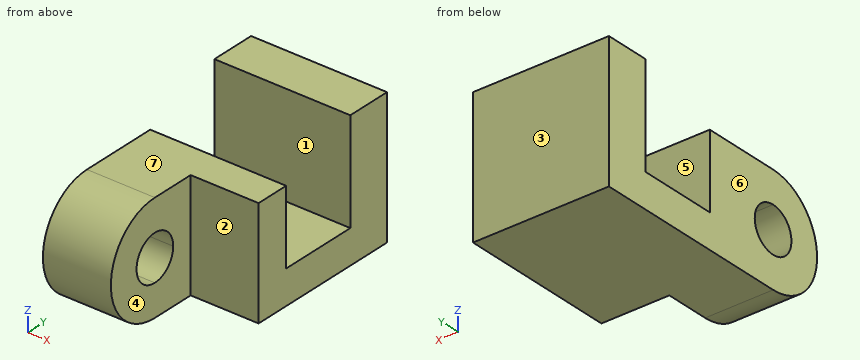
from build123d import *

# Parameters (mm, degrees)
F0_W      = 700
F0_H      = 600
F1_DEPTH  = 600
F3_DEPTH  = 600.001
F4_W      = 150
F4_H      = 120
F5_DEPTH  = 600.001
F6_W      = 300
F6_H      = 480
F7_DEPTH  = 195
F9_DEPTH  = 300
F11_DEPTH = 300.001


with BuildPart() as f1:
    # F0 (on Right) → F1 (new body)
    with BuildSketch(Plane.YZ):
        Rectangle(F0_W, F0_H)
    extrude(amount=F1_DEPTH)

    # F2 (on face) → F3 (cut, through all)
    with BuildSketch(Plane.YZ.offset(600)):
        Polygon((150, -150), (150, 300), (-200, 300), (-200, -150), (0, -150), align=None)
    extrude(amount=-F3_DEPTH, mode=Mode.SUBTRACT)

    # F4 (on face) → F5 (cut, through all)
    with BuildSketch(Plane.YZ.offset(600)):
        with Locations((-275, 240)):
            Rectangle(F4_W, F4_H)
    extrude(amount=-F5_DEPTH, mode=Mode.SUBTRACT)

    # F6 (on face) → F7 (join)
    with BuildSketch(Plane.XZ.offset(350)):
        with Locations((150, -60)):
            Rectangle(F6_W, F6_H)
    extrude(amount=F7_DEPTH)

    # F8 (on face) → F9 (join)
    with BuildSketch(Plane(origin=(0, 0, 0), x_dir=(0, -1, 0), z_dir=(-1, 0, 0))):
        with BuildLine():
            ThreePointArc((545, -300), (714.7056274848, -229.7056274848), (785, -60))
            ThreePointArc((785, -60), (714.7056274848, 109.7056274848), (545, 180))
            Line((545, 180), (545, -300))
        make_face()
    extrude(amount=-F9_DEPTH)

    # F10 (on face) → F11 (cut, through all)
    with BuildSketch(Plane.YZ.offset(300)):
        with BuildLine():
            ThreePointArc((-445, -60), (-474.2893218813, 10.7106781187), (-545, 40))
            Line((-545, 40), (-545, -160))
            ThreePointArc((-545, -160), (-474.2893218813, -130.7106781187), (-445, -60))
        make_face()
        with BuildLine():
            Line((-545, -160), (-545, 40))
            ThreePointArc((-545, 40), (-645, -60), (-545, -160))
        make_face()
    extrude(amount=-F11_DEPTH, mode=Mode.SUBTRACT)


solid = f1.part
Input: part model. Units: mm. Frame: model coordinates. Face numbers are marked on the shaded views. A direction names the side the tool comes from. Round coordinates to 2 decimals unless told otherwise and drop trailing zeros. Loops run counter-clockwise (first coordinate to the right, second up) from the corner with the lowest first, then second, coordinate; pieces in that order, holes last. Notation, with made-up numbers: (62, 14) -> (121, 14) arc R19 ccw to (121, 48) -> close; hole circle Ø5 at (1, -33). An arc over 180 degrees is marked (long way). Answer as a JSON object with one key per item and string values. Group by question number.
1) Section query B-B on y = -562. Output: boundary loops of the cut face in (x, z).
2) Ray query, L1, parallel to Y at x = 568, z = -86; L2, parallel to Y at x = 51.5, z = -122.5; L3, parallel to Y at x = 40, z = 30. Return the intervals inside material, ascending.
3) Draft query along Y for the marked faces 1, 2 and 3. Return one class per face: +Y half, -Y half, draft (parallel to the pull), parting line (faces both ways), or undercut.
4) Section query C-C on z = -124.5. Output: boundary loops of the cut face in (x, y), plus the area to 3 significant figures.
5) Section query A-A on x = 281.5. Output: boundary loops of the cut face in (y, z), plus the area to 3 significant figures.
6) Reachability of the marked faces 4, 5, 6 and 7 from +Z, -Z, +X, -X, +Y, -Y: full face, straight path, thin tool, end or side. Return the list, or none.
7) Section query D-D on z = 164.5. Output: boundary loops of the cut face in (x, y), plus the area to 3 significant figures.
8) Pin query (flat end, axial travel): pin 1 (6 mm diameter, centred on x = 354.5, z = -61.5, fed in from -Y); pin 2 (1 mm diameter, centred on y = -259, z = 151.5, fed in from -X); pin 3 (1.5 mm diameter, centred on x = 199, y = -248, fed in from +Z); pin 4 (2 mm diameter, centred on x = 312.5, y = -41, fed in from +Z). Return the tip coordinate at first contact, or that it passes through.
Reply:
{
 "1": {"outline": "(0, -299.4) -> (300, -299.4) -> (300, -158.54) -> (0, -158.54) -> close; (0, 38.54) -> (300, 38.54) -> (300, 179.4) -> (0, 179.4) -> close"},
 "2": {"L1": "y = -350 to -200, 150 to 350", "L2": "y = -776.72 to -623.06, -466.94 to -200, 150 to 350", "L3": "y = -767.49 to -588.59, -501.41 to -200, 150 to 350"},
 "3": {"face 1": "undercut", "face 2": "-Y half", "face 3": "+Y half"},
 "4": {"outline": "(0, -776.17) -> (300, -776.17) -> (300, -621.42) -> (0, -621.42) -> close; (0, -468.58) -> (300, -468.58) -> (300, -350) -> (600, -350) -> (600, -200) -> (0, -200) -> close; (0, 150) -> (600, 150) -> (600, 350) -> (0, 350) -> close", "area": "292,000 mm2"},
 "5": {"outline": "(-545, -300) -> (350, -300) -> (350, 300) -> (150, 300) -> (150, -150) -> (-200, -150) -> (-200, 180) -> (-545, 180) arc R240 ccw to start; hole circle Ø200 at (-545, -60)", "area": "397,000 mm2"},
 "6": {"face 4": "+Z, -Z, +X, -Y", "face 5": "+Z, +X, -X", "face 6": "+Z, -Z, -X, +Y, -Y", "face 7": "+Z, +X, -X, -Y"},
 "7": {"outline": "(0, -629.85) -> (300, -629.85) -> (300, -350) -> (600, -350) -> (600, -200) -> (0, -200) -> close; (0, 150) -> (600, 150) -> (600, 350) -> (0, 350) -> close", "area": "294,000 mm2"},
 "8": {"pin 1": "stops at y = -350", "pin 2": "stops at x = 0", "pin 3": "stops at z = 180", "pin 4": "stops at z = -150"}
}
